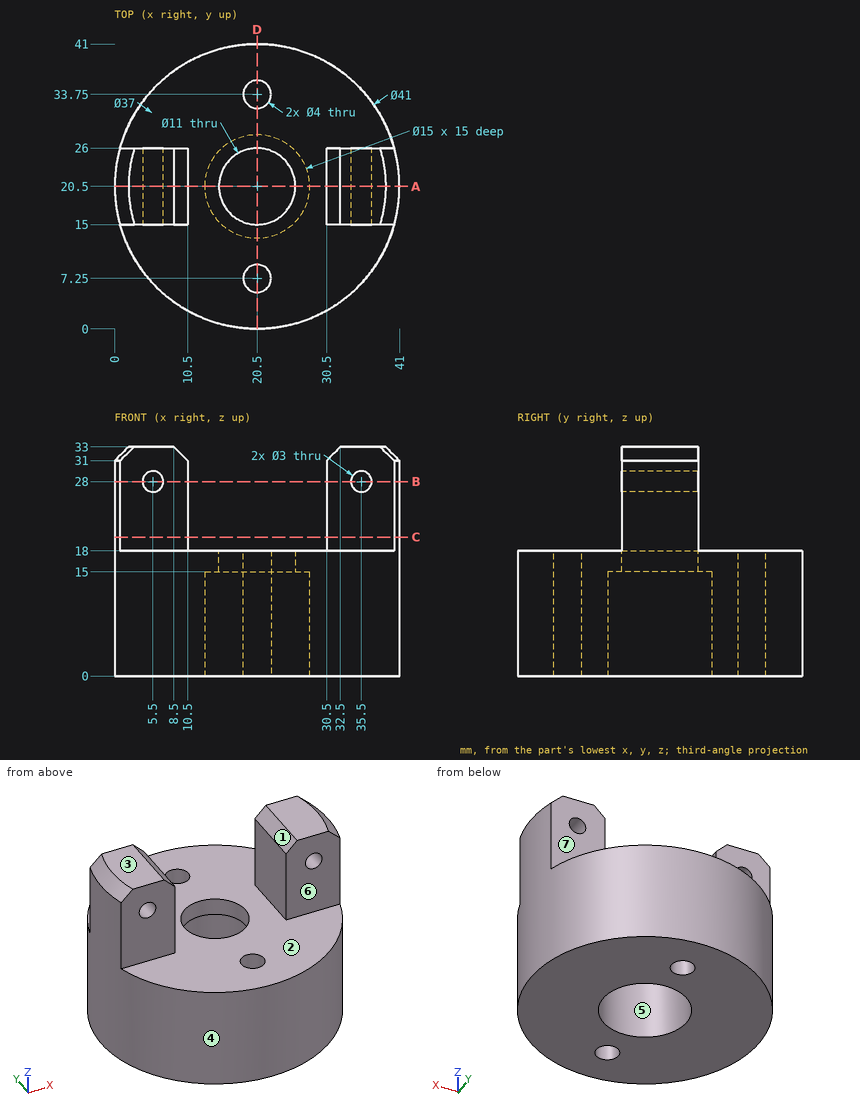
Geometry check sheet. Reference: drawing and pictorial views, mm from the part's lowest x, y, z. A direction names the side the tool comes from. Round coordinates to 2 decimals unless told otherwise and drop trailing zeros. Loops run counter-clockwise (first coordinate to the right, second up) from the corner with the lowest first, then second, coordinate; pieces in that order, holes last. Notation, with made-up numbers: (56, -3.75) - (70, -3.75) arc R23 cw to (70, 18.25) - close; hole circle Ø7 at (8, -12.5). An arc over 180 degrees is marked (long way). Use a Markdown table: item, result. Add a question column.
1. Access from +Z, -Z, +X, -X, +Y, -Y to the whole of each face (thin tool, end or side, straight path). Record for the marked faces 5, 6 and 7.
2. Section check D-D, the plane x = 20.5. Record the boundary of the cut face in (y, z), plus the area to 3 significant figures.
3. Release check for a two-part mould opening along X. For the marked faces 1, 2, 3 and 4 record: released by +X, released by -X, zero draft, split by the parting line, or undercut.
4. Section check C-C, the plane z = 20. Record the boundary of the cut face in (x, y), plus the area to 3 significant figures.
5. Section check B-B, the plane z = 28. Record the boundary of the cut face in (x, y), plus the area to 3 significant figures.
6. Gauge pin test, flat ends, axial feed: pin 1 (3 mm diameter, centred on x = 20.5, y = 33.75, fed in from -Z); pin 2 (5 mm diameter, centred on x = 5.5, z = 28, fed in from +Y); pin 3 (3 mm diameter, centred on x = 18, z = 4.5, fed in from +Y); pin 4 (8 mm diameter, centred on x = 9, z = 24.5, fed in from -Y). Record the tip position at first contact, or that the pin passes through.
7. Section check A-A, the plane y = 20.5. Record the boundary of the cut face in (x, z), plus the area to 3 significant figures.
8. Thickness scan on probe 1 along Y at (x, z) = (20.5, 6.75); probe 2 along Z at (x, y) = (5.5, 23.5); probe 3 along X at (y, z) = (16, 27). Record the ranges inside material, lowest first. Write a range as [from, to].
Checks:
| question | item | result |
|---|---|---|
| 1 | face 5 | -Z |
| 1 | face 6 | +Z, +X, -X, -Y |
| 1 | face 7 | +Z, +X, -X, +Y |
| 2 | outline | (0, 0) - (5.25, 0) - (5.25, 18) - (0, 18) - close; (9.25, 0) - (13, 0) - (13, 15) - (15, 15) - (15, 18) - (9.25, 18) - close; (26, 15) - (28, 15) - (28, 0) - (31.75, 0) - (31.75, 18) - (26, 18) - close; (35.75, 0) - (41, 0) - (41, 18) - (35.75, 18) - close |
| 2 | area | 336 mm^2 |
| 3 | face 1 | undercut |
| 3 | face 2 | undercut |
| 3 | face 3 | zero draft |
| 3 | face 4 | split by the parting line |
| 4 | outline | (0.75, 15) - (10.5, 15) - (10.5, 26) - (0.75, 26) arc R20.5 ccw to start; (30.5, 15) - (40.25, 15) arc R20.5 ccw to (40.25, 26) - (30.5, 26) - close |
| 4 | area | 226 mm^2 |
| 5 | outline | (0.75, 15) - (4, 15) - (4, 26) - (0.75, 26) arc R20.5 ccw to start; (7, 15) - (10.5, 15) - (10.5, 26) - (7, 26) - close; (30.5, 15) - (34, 15) - (34, 26) - (30.5, 26) - close; (37, 15) - (40.25, 15) arc R20.5 ccw to (40.25, 26) - (37, 26) - close |
| 5 | area | 160 mm^2 |
| 6 | pin 1 | passes through |
| 6 | pin 2 | stops at y = 26 |
| 6 | pin 3 | stops at y = 40.98 |
| 6 | pin 4 | stops at y = 15 |
| 7 | outline | (0, 0) - (13, 0) - (13, 15) - (15, 15) - (15, 18) - (10.5, 18) - (10.5, 31) - (8.5, 33) - (2, 33) - (0, 31) - close; (26, 15) - (28, 15) - (28, 0) - (41, 0) - (41, 31) - (39, 33) - (32.5, 33) - (30.5, 31) - (30.5, 18) - (26, 18) - close; hole circle Ø3 at (5.5, 28); hole circle Ø3 at (35.5, 28) |
| 7 | area | 773 mm^2 |
| 8 | probe 1 | y = [0, 5.25], [9.25, 13], [28, 31.75], [35.75, 41] |
| 8 | probe 2 | z = [0, 26.5], [29.5, 33] |
| 8 | probe 3 | x = [0.5, 4.38], [6.62, 10.5], [30.5, 34.38], [36.62, 40.5] |
